Geometry check sheet. Reference: the model listing, model coordinates, mm. A direction names the side the tool comes from. Give positions to 0.01 mm unless a question says otherwise; leave off trailing zeros. Write each loop counter-clockwise with the first axis right and the second up, starting at its lowest first coordinate (ties: lowest second). Pieces come first, ordered by that corner, then holes. Notation, with made-up numbers: (49, -20.5) - (92, -20.5) arc R27 cw to (92, 9.5) - close; hole circle Ø8 at (69.25, 59.5). An arc over 180 degrees is marked (long way). Use a Markdown table: item, result.
```python
from build123d import *

# Parameters (mm, degrees)
SKETCH1_R           = 1.7
BOSS_EXTRUDE1_DEPTH = 8.2
SKETCH2_W           = 29
SKETCH2_H           = 10
BOSS_EXTRUDE2_DEPTH = 8.2
FILLET2_R           = 1
FILLET3_R           = 2


with BuildPart() as part:
    # Sketch1 → Boss-Extrude1 (new body)
    with BuildSketch(Plane.XY):
        with BuildLine():
            Line((-21.15, 14.65), (-21.15, -14.65))
            ThreePointArc((-21.15, -14.65), (-20.891190411, -15.95112367), (-20.154163056, -17.054163056))
            Line((-20.154163056, -17.054163056), (-17.054163056, -20.154163056))
            ThreePointArc((-17.054163056, -20.154163056), (-15.95112367, -20.891190411), (-14.65, -21.15))
            Line((-14.65, -21.15), (14.65, -21.15))
            ThreePointArc((14.65, -21.15), (15.95112367, -20.891190411), (17.054163056, -20.154163056))
            Line((17.054163056, -20.154163056), (20.154163056, -17.054163056))
            ThreePointArc((20.154163056, -17.054163056), (20.891190411, -15.95112367), (21.15, -14.65))
            Line((21.15, -14.65), (21.15, 14.65))
            ThreePointArc((21.15, 14.65), (20.891190411, 15.95112367), (20.154163056, 17.054163056))
            Line((20.154163056, 17.054163056), (17.054163056, 20.154163056))
            ThreePointArc((17.054163056, 20.154163056), (15.95112367, 20.891190411), (14.65, 21.15))
            Line((14.65, 21.15), (-14.65, 21.15))
            ThreePointArc((-14.65, 21.15), (-15.95112367, 20.891190411), (-17.054163056, 20.154163056))
            Line((-17.054163056, 20.154163056), (-20.154163056, 17.054163056))
            ThreePointArc((-20.154163056, 17.054163056), (-20.891190411, 15.95112367), (-21.15, 14.65))
        make_face()
        with Locations((-15.5, 15.5)):
            Circle(SKETCH1_R, mode=Mode.SUBTRACT)
        with Locations((15.5, 15.5)):
            Circle(SKETCH1_R, mode=Mode.SUBTRACT)
        with Locations((15.5, -15.5)):
            Circle(SKETCH1_R, mode=Mode.SUBTRACT)
        with Locations((-15.5, -15.5)):
            Circle(SKETCH1_R, mode=Mode.SUBTRACT)
    extrude(amount=BOSS_EXTRUDE1_DEPTH)

    # Sketch2 → Boss-Extrude2 (add)
    with BuildSketch(Plane.XY.offset(8.2)):
        with Locations((0, 6.849045043)):
            Rectangle(SKETCH2_W, SKETCH2_H)
    extrude(amount=BOSS_EXTRUDE2_DEPTH)

    # Fillet2
    fillet2_edges = [part.edges().sort_by_distance(p)[0] for p in [
        (15.95112367, 20.891190411, 8.2),
        (0, 21.15, 8.2),
        (-15.95112367, 20.891190411, 8.2),
        (-18.604163056, 18.604163056, 8.2),
        (-20.891190411, 15.95112367, 8.2),
        (-21.15, 0, 8.2),
        (-20.891190411, -15.95112367, 8.2),
        (-18.604163056, -18.604163056, 8.2),
        (-15.95112367, -20.891190411, 8.2),
        (0, -21.15, 8.2),
        (20.891190411, 15.95112367, 8.2),
        (15.95112367, -20.891190411, 8.2),
        (18.604163056, -18.604163056, 8.2),
        (20.891190411, -15.95112367, 8.2),
        (21.15, 0, 8.2),
        (-14.5, 6.849045043, 16.4),
        (0, 1.849045043, 16.4),
        (14.5, 6.849045043, 16.4),
        (0, 11.849045043, 16.4),
        (18.604163056, 18.604163056, 8.2),
    ]]
    fillet(fillet2_edges, radius=FILLET2_R)

    # Fillet3
    # the kernel refuses this fillet: 2 mm, written as the material it takes off along each edge
    with BuildSketch(Plane(origin=(12.5, 3.849045043, 16.4), x_dir=(0, -1, 0), z_dir=(-1, 0, 0))) as fillet3_piece_1:
        with BuildLine():
            CenterArc((1, -1), 1, 0, 90)
            Line((2, -1), (2, 0))
            Line((2, 0), (1, 0))
        make_face()
    revolve(axis=Axis((12.5, 3.849045043, 16.4), (0, 0, 1)), revolution_arc=90, mode=Mode.SUBTRACT)
    with BuildSketch(Plane(origin=(-12.5, 3.849045043, 16.4), x_dir=(-1, 0, 0), z_dir=(0, 1, 0))) as fillet3_piece_2:
        with BuildLine():
            CenterArc((1, -1), 1, 0, 90)
            Line((2, -1), (2, 0))
            Line((2, 0), (1, 0))
        make_face()
    revolve(axis=Axis((-12.5, 3.849045043, 16.4), (0, 0, 1)), revolution_arc=90, mode=Mode.SUBTRACT)
    with BuildSketch(Plane(origin=(12.5, 9.849045043, 16.4), x_dir=(1, 0, 0), z_dir=(0, -1, 0))) as fillet3_piece_3:
        with BuildLine():
            CenterArc((1, -1), 1, 0, 90)
            Line((2, -1), (2, 0))
            Line((2, 0), (1, 0))
        make_face()
    revolve(axis=Axis((12.5, 9.849045043, 16.4), (0, 0, 1)), revolution_arc=90, mode=Mode.SUBTRACT)
    with BuildSketch(Plane(origin=(-12.5, 9.849045043, 16.4), x_dir=(0, 1, 0), z_dir=(1, 0, 0))) as fillet3_piece_4:
        with BuildLine():
            CenterArc((1, -1), 1, 0, 90)
            Line((2, -1), (2, 0))
            Line((2, 0), (1, 0))
        make_face()
    revolve(axis=Axis((-12.5, 9.849045043, 16.4), (0, 0, 1)), revolution_arc=90, mode=Mode.SUBTRACT)
    with BuildSketch(Plane(origin=(-14.5, 11.849045043, 8.2), x_dir=(0, -1, 0), z_dir=(0, 0, 1))) as fillet3_piece_5:
        with BuildLine():
            CenterArc((FILLET3_R, FILLET3_R), FILLET3_R, 180, 90)
            Line((0, FILLET3_R), (0, 0))
            Line((0, 0), (FILLET3_R, 0))
        make_face()
    extrude(amount=8.2, mode=Mode.SUBTRACT)
    with BuildSketch(Plane(origin=(14.5, 11.849045043, 8.2), x_dir=(0, -1, 0), z_dir=(0, 0, 1)), Plane(origin=(14.5, 1.849045043, 8.2), x_dir=(-1, 0, 0), z_dir=(0, 0, 1)), Plane(origin=(-14.5, 1.849045043, 8.2), x_dir=(0, 1, 0), z_dir=(0, 0, 1))) as fillet3_piece_6:
        with BuildLine():
            CenterArc((FILLET3_R, -FILLET3_R), FILLET3_R, 90, 90)
            Line((0, -FILLET3_R), (0, 0))
            Line((0, 0), (FILLET3_R, 0))
        make_face()
    extrude(amount=8.2, mode=Mode.SUBTRACT)


solid = part.part
```
1) Material ranges on L1, parallel to Y at x = 16, z = 6.75; L2, parallel to Y at x = -1, z = 10.75; L3, parallel to Z at x = -2.5, y = -1, recorded low to high. Write a range as from..to.
Working result:
| item | result |
|---|---|
| L1 | y = -20.87..-17.12, -13.88..13.88, 17.12..20.87 |
| L2 | y = 1.85..11.85 |
| L3 | z = 0..8.2 |
2) Section check A-A on x = -10.5. Record the boundary of the cut face in (y, z).
Working result:
| item | result |
|---|---|
| outline | (-21.15, 0) - (21.15, 0) - (21.15, 7.2) arc R1 ccw to (20.15, 8.2) - (11.85, 8.2) - (11.85, 15.4) arc R1 ccw to (10.85, 16.4) - (2.85, 16.4) arc R1 ccw to (1.85, 15.4) - (1.85, 8.2) - (-20.15, 8.2) arc R1 ccw to (-21.15, 7.2) - close |
3) Section check C-C on y = 15.5. Count the separate pieces of the cut face and the enclosed holes in it, then the cut area to 3 significant figures.
Working result:
| item | result |
|---|---|
| separate pieces | 3 |
| enclosed holes | 0 |
| area | 289 mm² |
4) Mould release check, pull along Y, two halves, no side actions. Record for faces 4 (the flat face through (18.58, -18.63, 3.55)), 5 (the cylindrical face through (-15.93, 20.9, 3.55)), 6 (the cylindrical face through (14.215, 6.891, 16.099)), 7 (the cylindrical face through (-13.93, -16.15, 4.04)): pulls with the +Y half, pulls with the -Y half, needs draft (parallel to the pull), parting line crosses it, or undercut.
Working result:
| item | result |
|---|---|
| face 4 | pulls with the -Y half |
| face 5 | pulls with the +Y half |
| face 6 | needs draft |
| face 7 | undercut |
5) Set-up check for faces 1 (the flat face through (14.5, 7, 12)), 2 (the cylindrical face through (13.9, 2.42, 11.75)), 3 (the cylindrical face through (-20.849, -0.205, 7.915)): record each of +Z, -Z, +X, -X, +Y, -Y from which the full face is reachable in a straight line by a thin tool's end or side.
Working result:
| item | result |
|---|---|
| face 1 | +Z, +X, +Y, -Y |
| face 2 | +Z, +X, -Y |
| face 3 | +Z, -X, +Y, -Y |
6) Depth check by flat-ended pin: P1, Ø1.5, axis at x = 16, y = 2.5, coming from the +Z side; P2, Ø6.5, axis at y = 6, z = 12, coming from the -X side; P3, Ø3, axis at x = -15.5, y = 15.5, coming from the -Z side; P4, Ø1.8, axis at y = 7, z = 12, coming from the +X side. Enter the tip coordinate at first touch or a pass-through.
Working result:
| item | result |
|---|---|
| P1 | stops at z = 8.2 |
| P2 | stops at x = -14.5 |
| P3 | passes through |
| P4 | stops at x = 14.5 |
7) Section check B-B on y = -4. Record the boundary of the cut face in (x, z), then the cut area to 3 significant figures.
Working result:
| item | result |
|---|---|
| outline | (-21.15, 0) - (21.15, 0) - (21.15, 7.2) arc R1 ccw to (20.15, 8.2) - (-20.15, 8.2) arc R1 ccw to (-21.15, 7.2) - close |
| area | 346 mm² |
